The model under review builds one solid part; all positions refer to its coordinate system, in mm. A direction names the side the tool comes from. Round coordinates to 2 decimals unless told otherwise and drop trailing zeros. Loops run counter-clockwise (first coordinate to the right, second up) from the corner with the lowest first, then second, coordinate; pieces in that order, holes last. Notation, with made-up numbers: (-40, 86) -> (13, 86) arc R17 cw to (13, 97) -> close; hole circle Ø1 at (11, -35.5). An arc over 180 degrees is marked (long way). Use a Markdown table: item, result. Add a question column.
1) Insertion check: pin 1 (1 mm diameter, centred on x = 41.5, y = -615.5, fed in from -Z); pin 2 (5 mm diameter, centred on x = 35, y = -276.5, fed in from +Z); pin 3 (3 mm diameter, centred on y = -1614.5, z = -5.5, fed in from -X). Each pin has a flat end and moves straight along its axis. Give the tip position at first contact, or say it passes through.
2) For faces 1 (the cylindrical face through (-99.903, -986, 4.397)), 2 (the cylindrical face through (-101.488, -1950.916, -1.587)), list the 3-axis set-ups (+Z, -Z, +X, -X, +Y, -Y) from which the entire face can be reached by the end or side of a thin tool; tool diameter is ignored.
3) Consider section A-A on y = -1752.5. Give the boundary of the cut face in (x, z), plus the area to 3 significant figures.
4) Mouldability with a two-part tool opening along Z and no side actions: class faces 3 (the flat face through (101, -1957, 0)), 4 (the flat face through (-16, 0, 100)), 5 (the cylindrical face through (-102.9, -986, 4.5)) as released by +Z, released by -Z, zero draft, split by the parting line, or undercut.
5) Consider section B-B on z = 0. Give the boundary of the cut face in (x, y).
6) Wall thickness on probe 1 along X at (y, z) = (-1078.5, 0); probe 2 along X at (y, z) = (-1192, 7.5): over which ranges is each line inside the solid? List them lowest first.
7) Consider section C-C on x = 0. Give the boundary of the cut face in (y, z), plus the area to 3 significant figures.
8) Consider section D-D on y = -418. Give the boundary of the cut face in (x, z).
from build123d import *

# Parameters (mm, degrees)
F0_R     = 103
F0_R_2   = 100
F1_DEPTH = 2000
F4_DEPTH = 240
F6_DEPTH = 12


with BuildPart() as f1:
    # F0 (on Front) → F1 (new body)
    with BuildSketch(Plane.XZ):
        Circle(F0_R)
        Circle(F0_R_2, mode=Mode.SUBTRACT)
    extrude(amount=F1_DEPTH)

    # F3 (on offset) → F4 (cut)
    with BuildSketch(Plane.XZ.offset(1945)):
        with BuildLine():
            Line((14.631978, -30), (45.590599, -93.474581))
            ThreePointArc((45.590599, -93.474581), (104, 0), (45.590599, 93.474581))
            Line((45.590599, 93.474581), (15.458162, 31.693928))
            Line((15.458162, 31.693928), (-15.458162, 31.693928))
            Line((-15.458162, 31.693928), (-45.590599, 93.474581))
            ThreePointArc((-45.590599, 93.474581), (-104, 0), (-45.590599, -93.474581))
            Line((-45.590599, -93.474581), (-14.631978, -30))
            Line((-14.631978, -30), (14.631978, -30))
        make_face()
    extrude(amount=-F4_DEPTH, mode=Mode.SUBTRACT)

    # F5 (on face) → F6 (cut)
    with BuildSketch(Plane(origin=(0, -1945, 0), x_dir=(-1, 0, 0), z_dir=(0, 1, 0))):
        with BuildLine():
            Line((-44.494671, -91.227596), (-7.343568, -15.056546))
            Line((-7.343568, -15.056546), (-7.343568, 15.056546))
            Line((-7.343568, 15.056546), (-44.494671, 91.227596))
            ThreePointArc((-44.494671, 91.227596), (-101.5, 0), (-44.494671, -91.227596))
        make_face()
        with BuildLine():
            Line((7.343568, 15.056546), (7.343568, -15.056546))
            Line((7.343568, -15.056546), (44.494671, -91.227596))
            ThreePointArc((44.494671, -91.227596), (101.5, 0), (44.494671, 91.227596))
            Line((44.494671, 91.227596), (7.343568, 15.056546))
        make_face()
    extrude(amount=-F6_DEPTH, mode=Mode.SUBTRACT)


solid = f1.part
Result set:
| question | item | result |
|---|---|---|
| 1 | pin 1 | z = -94.49 |
| 1 | pin 2 | z = 97.74 |
| 1 | pin 3 | x = -102.92 |
| 2 | face 1 | +Y, -Y |
| 2 | face 2 | none |
| 3 | outline | (-45.15, -92.58) arc R103 ccw to (45.15, -92.58) -> (43.84, -89.88) arc R100 cw to (-43.84, -89.88) -> close; (-45.15, 92.58) -> (-43.84, 89.88) arc R100 cw to (43.84, 89.88) -> (45.15, 92.58) arc R103 ccw to start |
| 3 | area | 553 mm2 |
| 4 | face 3 | undercut |
| 4 | face 4 | zero draft |
| 4 | face 5 | split by the parting line |
| 5 | outline | (-103, -2000) -> (-100, -2000) -> (-100, -1957) -> (-101.5, -1957) -> (-101.5, -1945) -> (-103, -1945) -> close; (-103, -1705) -> (-100, -1705) -> (-100, 0) -> (-103, 0) -> close; (100, -2000) -> (103, -2000) -> (103, -1945) -> (101.5, -1945) -> (101.5, -1957) -> (100, -1957) -> close; (100, -1705) -> (103, -1705) -> (103, 0) -> (100, 0) -> close |
| 6 | probe 1 | -103 to -100, 100 to 103 |
| 6 | probe 2 | -102.73 to -99.72, 99.72 to 102.73 |
| 7 | outline | (-2000, -103) -> (0, -103) -> (0, -100) -> (-2000, -100) -> close; (-2000, 100) -> (0, 100) -> (0, 103) -> (-2000, 103) -> close |
| 7 | area | 12,000 mm2 |
| 8 | outline | circle Ø206 at (0, 0); hole circle Ø200 at (0, 0) |
